```python
from build123d import *

# Parameters (mm, degrees)
F0_R          = 25
F0_W          = 25.4
F0_H          = 25.4
F1_DEPTH      = 2
F2_R          = 2
F3_DEPTH      = 2.5
F3_DEPTH_BACK = 2.5
F4_SIZE       = 0.5
F5_R          = 0.99999
F6_T4_DEPTH   = 5
F6_T9_DEPTH   = 5.1486606532
F6_T15_DEPTH  = 5.1486606532
F6_T18_DEPTH  = 20
F6_T20_DEPTH  = 14.2973213065


# Not quite as in the source:
# - a fillet or chamfer that OpenCascade refuses, or shapes differently, is made with other operations: its cross-section is extruded or revolved along the edge and cut away or added
# - a fillet or chamfer is up to 0.001 mm smaller than in the source, because OpenCascade refuses the exact size


with BuildPart() as f1:
    # F0 (on Top) → F1 (new body)
    with BuildSketch(Plane.XY):
        Circle(F0_R)
        Rectangle(F0_W, F0_H, mode=Mode.SUBTRACT)
    extrude(amount=F1_DEPTH)

    # F2 (on Front) → F3 (join, two sides)
    with BuildSketch(Plane.XZ) as f3_sk:
        Polygon((-24, 10), (-24, 1.4085747534), (-14.7320097312, 1.4085747534), (-19, 10), align=None)
        with Locations((-21, 6)):
            Circle(F2_R, mode=Mode.SUBTRACT)
    extrude(amount=F3_DEPTH)
    extrude(f3_sk.sketch, amount=-F3_DEPTH_BACK)

    # F4
    f4_edges = [f1.edges().sort_by_distance(p)[0] for p in [
        (0, 12.7, 2),
        (12.7, 0, 2),
        (0, -12.7, 2),
        (-12.7, 0, 2),
        (-25, 0, 2),
        (-19.512907, 2.5, 2),
        (-19.512907, -2.5, 2),
    ]]
    chamfer(f4_edges, length=F4_SIZE)

    # F5 (radius 1 in the source; OpenCascade refuses exactly that, so slightly less here)
    f5_edges = [f1.edges().sort_by_distance(p)[0] for p in [
        (-23, -2.5, 6),
        (-23, 2.5, 6),
    ]]
    fillet(f5_edges, radius=F5_R)

    # F6: fillet of radius 3 on 3 edges, made by hand


with BuildPart() as f6_tool2:
    # F6_s3 → F6_t4 (new body)
    with BuildSketch(Plane.XZ.offset(-2.5)):
        with BuildLine():
            ThreePointArc((-15.8530900959, 3.66529924), (-14.7468397832, 2.4500880133), (-13.1663497137, 2))
            Line((-13.1663497137, 2), (-15.025813975, 2))
            Line((-15.025813975, 2), (-15.8530900959, 3.66529924))
        make_face()
    extrude(amount=F6_T4_DEPTH)

    split(bisect_by=Plane(origin=(-5.6, 0, -5.6), x_dir=(0, 1, 0), z_dir=(-0.7071067812, 0, -0.7071067812)), keep=Keep.TOP)


with BuildPart() as f1_1:
    add(f1.part)

    # F6_t1: union F6_tool2
    add(f6_tool2.part)


with BuildPart() as f6_tool7:
    # F6_s8 → F6_t9 (new body)
    with BuildSketch(Plane.XZ.offset(-2.5)):
        with BuildLine():
            ThreePointArc((-15.8530900959, 3.66529924), (-14.7468397832, 2.4500880133), (-13.1663497137, 2))
            Line((-13.1663497137, 2), (-15.025813975, 2))
            Line((-15.025813975, 2), (-15.8530900959, 3.66529924))
        make_face()
    extrude(amount=-F6_T9_DEPTH)

    split(bisect_by=Plane(origin=(0, 2.5, 2.5), x_dir=(1, 0, 0), z_dir=(0, -0.7071067812, -0.7071067812)), keep=Keep.TOP)

    split(bisect_by=Plane(origin=(-5.6, 0, -5.6), x_dir=(0, 1, 0), z_dir=(-0.7071067812, 0, -0.7071067812)), keep=Keep.TOP)


with BuildPart() as f1_2:
    add(f1_1.part)

    # F6_t6: union F6_tool7
    add(f6_tool7.part)


with BuildPart() as f6_tool13:
    # F6_s14 → F6_t15 (new body)
    with BuildSketch(Plane.XZ.offset(2.5)):
        with BuildLine():
            ThreePointArc((-15.8530900959, 3.66529924), (-14.7468397832, 2.4500880133), (-13.1663497137, 2))
            Line((-13.1663497137, 2), (-15.025813975, 2))
            Line((-15.025813975, 2), (-15.8530900959, 3.66529924))
        make_face()
    extrude(amount=F6_T15_DEPTH)

    split(bisect_by=Plane(origin=(0, -2.5, 2.5), x_dir=(1, 0, 0), z_dir=(0, 0.7071067812, -0.7071067812)), keep=Keep.TOP)

    split(bisect_by=Plane(origin=(-5.6, 0, -5.6), x_dir=(0, 1, 0), z_dir=(-0.7071067812, 0, -0.7071067812)), keep=Keep.TOP)


with BuildPart() as f1_3:
    add(f1_2.part)

    # F6_t12: union F6_tool13
    add(f6_tool13.part)

    # F6_s19 → F6_t18 (cut)
    with BuildSketch(Plane.XZ.offset(-10)):
        with BuildLine():
            ThreePointArc((-24, 7), (-23.1213203436, 9.1213203436), (-21, 10))
            Line((-21, 10), (-24, 10))
            Line((-24, 10), (-24, 7))
        make_face()
    extrude(amount=F6_T18_DEPTH, mode=Mode.SUBTRACT)

    # F6_s21 → F6_t20 (cut)
    with BuildSketch(Plane.XZ.offset(-7.1486606532)):
        with BuildLine():
            ThreePointArc((-20.8594642613, 10), (-19.2789741917, 9.5499119867), (-18.1727238791, 8.33470076))
            Line((-18.1727238791, 8.33470076), (-19, 10))
            Line((-19, 10), (-20.8594642613, 10))
        make_face()
    extrude(amount=F6_T20_DEPTH, mode=Mode.SUBTRACT)


solid = f1_3.part
```
Design review of the part built by this model. Coordinates are the model's own, in mm. A direction names the side the tool comes from. Give positions to 0.01 mm unless a question says otherwise; leave off trailing zeros. Write each loop counter-clockwise with the first axis right and the second up, starting at its lowest first coordinate (ties: lowest second). Pieces come first, ordered by that corner, then holes. Notation, with made-up numbers: (48.25, 73) - (73.25, 73) arc R21 ccw to (73.25, 104) - close; hole circle Ø10 at (-13.75, 12.5). An arc over 180 degrees is marked (long way). Return JSON: item names as keys, results as strings. Group by question number.
(1) Insertion check: pin 1 (5 mm diameter, centred on x = 19, z = 4, fed in from +Y); pin 2 (1.2 mm diameter, centred on y = 3, z = 0.5, fed in from +X); pin 3 (2.5 mm diameter, centred on x = -19.5, z = 7, fed in from +Y); pin 4 (6 mm diameter, centred on x = -8, z = 7, fed in from +Y). Each pin has a flat end and moves straight along its axis. Give the tip position at first contact, or say it passes through.
(2) To check wall thickness, follow probe 1 along Z at (x, y) = (-21, 0); probe 2 along Z at (x, y) = (-12.5, -18); probe 3 along Y at (x, z) = (-18, 2.75). State the ranges of each line that lie inside material, in increasing order.
(3) We need section B-B, the plane x = 0. Give the boundary of the cut face in (y, z).
(4) Mouldability with a two-part tool opening along Y and no side actions: class faces 1 (the flat face through (-18, 2.5, 5)), 2 (the cylindrical face through (-14.78, 0.04, 2.47)), 3 (the flat face through (-12.7, 0, 1)) as +Y half, -Y half, draft (parallel to the pull), parting line (faces both ways), or undercut.
(5) We need section A-A, the plane y = 0. Give the boundary of the cut face in (x, z).
(6) Machinability: for faces 4 (the flat face through (12.7, 0, 1)), 5 (the flat face through (-24, 0, 5)), 6 (the flat face through (-18, -2.5, 5)), which of the approach directions +Z, -Z, +X, -X, +Y, -Y give a long, thin tool a straight path to every point of the face, cutting with its end or side? Answer none if there is none.
Reported:
{
 "1": {"pin 1": "stops at y = 17.15", "pin 2": "stops at x = 24.88", "pin 3": "stops at y = 2.5", "pin 4": "passes through"},
 "2": {"probe 1": "z = 0 to 4, 8 to 10", "probe 2": "z = 0 to 2", "probe 3": "y = -2.5 to 2.5"},
 "3": {"outline": "(-25, 0) - (-12.7, 0) - (-12.7, 1.5) - (-13.2, 2) - (-24.5, 2) - (-25, 1.5) - close; (12.7, 0) - (25, 0) - (25, 1.5) - (24.5, 2) - (13.2, 2) - (12.7, 1.5) - close"},
 "4": {"face 1": "+Y half", "face 2": "draft", "face 3": "undercut"},
 "5": {"outline": "(-25, 0) - (-12.7, 0) - (-12.7, 1.5) - (-13.2, 2) arc R3 cw to (-15.85, 3.67) - (-18.17, 8.33) arc R3 ccw to (-20.86, 10) - (-21, 10) arc R3 ccw to (-24, 7) - (-24, 2) - (-24.5, 2) - (-25, 1.5) - close; (12.7, 0) - (25, 0) - (25, 1.5) - (24.5, 2) - (13.2, 2) - (12.7, 1.5) - close; hole circle Ø4 at (-21, 6)"},
 "6": {"face 4": "+Z, -Z", "face 5": "+Z, -X, +Y, -Y", "face 6": "+Z, +X, -X, -Y"}
}
